```python
from build123d import *

# Parameters (mm, degrees)
F0_W     = 177.8
F0_H     = 76.2
F1_DEPTH = 25.4
F2_DEPTH = 101.6


with BuildPart() as f1:
    # F0 (on Front) → F1 (new body)
    with BuildSketch(Plane.XZ):
        with Locations((3.457811, 0.322963)):
            Rectangle(F0_W, F0_H)
    extrude(amount=F1_DEPTH)

    # F0 (on Front) → F2 (join)
    with BuildSketch(Plane.XZ):
        Polygon((-85.442189, 63.817453), (-85.442189, 38.422963), (92.357811, 38.422963), (91.828754, 63.817453), align=None)
    extrude(amount=F2_DEPTH)


solid = f1.part
```
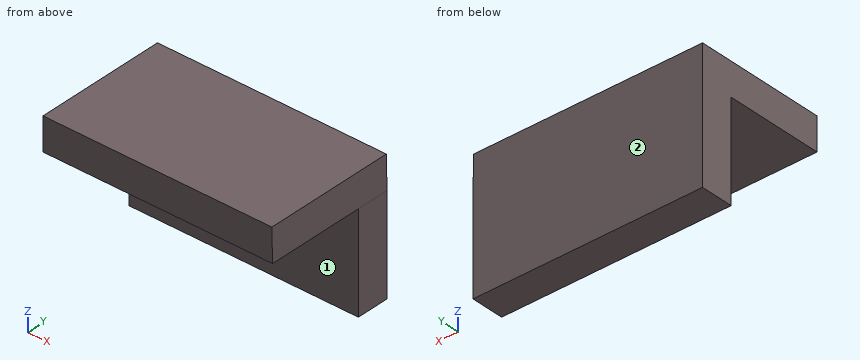
The listing builds one solid part. Answer for the finished solid, in the listing's coordinates (mm). Face numbers are marked on the shaded views. A direction names the side the tool comes from. Give positions to 0.01 mm unless a question says otherwise; leave off trailing zeros. Loops run counter-clockwise (first coordinate to the right, second up) from the corner with the lowest first, then second, coordinate; pieces in that order, holes last. Notation, with made-up numbers: (-9, 5.5) - (4, 5.5) arc R19 cw to (4, 40.5) - close; hole circle Ø1 at (2, 43.25). An arc over 180 degrees is marked (long way). Return JSON: item names as keys, results as strings. Group by question number.
1. Given pin 1 Ø3 at (x, z) = (10.5, 16) entering from -Y; pin 2 Ø10 at (x, y) = (-66, -63) entering from -Z, each flat-ended and moving along its own axis, determine where each tip first touches the part or whether it passes through.
2. Find section B-B (y = -46). Write down the section's boundary in (x, z).
3. Find section C-C (x = -9.5). Write down the section's boundary in (y, z).
4. Straight lines are drawn through the part: line 1 (Z direction, x = -51, y = -90); line 2 (Y direction, x = 23, z = 35); line 3 (X direction, y = -92.5, z = 57.5). For each, find the intervals that lie inside material, in ascending order. Write a range as [from, to].
5. Which of the six approach directions +Z, -Z, +X, -X, +Y, -Y give full straight-line access (tool end or side, diameter ignored) to the marked faces 1 and 2?
6. Find section A-A (z = -20). Write down the section's boundary in (x, y), then the cut area to 3 significant figures.
Verdict:
{
 "1": {"pin 1": "stops at y = -25.4", "pin 2": "stops at z = 38.42"},
 "2": {"outline": "(-85.44, 38.42) - (92.36, 38.42) - (91.83, 63.82) - (-85.44, 63.82) - close"},
 "3": {"outline": "(-101.6, 38.42) - (-25.4, 38.42) - (-25.4, -37.78) - (0, -37.78) - (0, 63.82) - (-101.6, 63.82) - close"},
 "4": {"line 1": "z = [38.42, 63.82]", "line 2": "y = [-25.4, 0]", "line 3": "x = [-85.44, 91.96]"},
 "5": {"face 1": "-Z, +X, -X, -Y", "face 2": "+Z, -Z, +X, -X, +Y"},
 "6": {"outline": "(-85.44, -25.4) - (92.36, -25.4) - (92.36, 0) - (-85.44, 0) - close", "area": "4,520 mm^2"}
}
